The listing builds one solid part. Answer for the finished solid, in the listing's coordinates (mm). A direction names the side the tool comes from. Give positions to 0.01 mm unless a question says otherwise; leave off trailing zeros. Order: outer loops, then holes, each group sorted by start corner. A loop starts at its lowest first (then second) coordinate and runs counter-clockwise, first axis right, second up. Notation, with made-up numbers: (31.25, 76) - (68.25, 76) arc R15 ccw to (68.25, 87) - close; hole circle Ø5 at (1.5, -20). An arc over 180 degrees is marked (long way). Answer in a Markdown table with one row per item. Add a question column.
```python
from build123d import *

# Parameters (mm, degrees)
SKETCH1_W                                        = 22.225
SKETCH1_H                                        = 25.4
EXTRUDE1_DEPTH                                   = 12.7
SKETCH2_W                                        = 9.525
SKETCH2_H                                        = 0.762
EXTRUDE2_DEPTH                                   = 25.4
SKETCH3_W                                        = 0.762
SKETCH3_H                                        = 13.678822609
EXTRUDE3_DEPTH                                   = 25.4
EXTRUDE4_DEPTH                                   = 25.4
SKETCH7_W                                        = 3.175
SKETCH7_H                                        = 25.4
EXTRUDE5_DEPTH                                   = 6.74624
SKETCH8_W                                        = 15.875
SKETCH8_H                                        = 15.875
EXTRUDE6_DEPTH                                   = 25.4
F_1_4_20_TAPPED_HOLE1_D                          = 5.1054
F_1_4_20_TAPPED_HOLE1_DEPTH                      = 9.525
F_1_4_20_TAPPED_HOLE1_TIP                        = 1.533816902
EXTRUDE7_DEPTH                                   = 53.055785583
SKETCH10_W                                       = 9.525
SKETCH10_H                                       = 7.700729076
EXTRUDE8_DEPTH                                   = 25.4
CBORE_FOR_1_4_SOCKET_HEAD_CAP_SCREW1_D           = 6.7564
CBORE_FOR_1_4_SOCKET_HEAD_CAP_SCREW1_DEPTH       = 9.525
CBORE_FOR_1_4_SOCKET_HEAD_CAP_SCREW1_CBORE_D     = 11.1125
CBORE_FOR_1_4_SOCKET_HEAD_CAP_SCREW1_CBORE_DEPTH = 6.35
F_1_4_20_TAPPED_HOLE2_D                          = 5.1054
FILLET1_R                                        = 1.5875
FILLET2_R                                        = 7.9375


with BuildPart() as part:
    # Sketch1 → Extrude1 (new, symmetric)
    with BuildSketch(Plane.XY):
        Rectangle(SKETCH1_W, SKETCH1_H)
        Polygon((0, 10.998522628), (-9.525, 5.499261314), (-9.525, -5.499261314), (0, -10.998522628), (9.525, -5.499261314), (9.525, 5.499261314), align=None, mode=Mode.SUBTRACT)
    extrude(amount=EXTRUDE1_DEPTH, both=True)

    # Sketch2 → Extrude2 (add)
    with BuildSketch(Plane.XY.offset(12.7)):
        with Locations((15.875, 5.969)):
            Rectangle(SKETCH2_W, SKETCH2_H)
        with Locations((15.875, -3.772822609)):
            Rectangle(SKETCH2_W, SKETCH2_H)
        with Locations((-15.875, -3.772822609)):
            Rectangle(SKETCH2_W, SKETCH2_H)
        with Locations((-15.875, 5.969)):
            Rectangle(SKETCH2_W, SKETCH2_H)
    extrude(amount=-EXTRUDE2_DEPTH)

    # Sketch3 → Extrude3 (add)
    with BuildSketch(Plane.XY.offset(12.7)):
        with Locations((21.0185, 2.685588695)):
            Rectangle(SKETCH3_W, SKETCH3_H)
        with Locations((-21.0185, 2.685588695)):
            Rectangle(SKETCH3_W, SKETCH3_H)
    extrude(amount=-EXTRUDE3_DEPTH)

    # Sketch4 → Extrude4 (add)
    with BuildSketch(Plane.XY.offset(12.7)):
        Polygon((-21.3995, 17.4625), (21.3995, 17.4625), (21.3995, 9.525), (14.2875, 9.525), (14.2875, 15.875), (-14.2875, 15.875), (-14.2875, 9.525), (-21.3995, 9.525), align=None)
    extrude(amount=-EXTRUDE4_DEPTH)

    # Sketch7 → Extrude5 (add)
    with BuildSketch(Plane(origin=(0, 17.4625, 0), x_dir=(1, 0, 0), z_dir=(0, 1, 0))):
        Rectangle(SKETCH7_W, SKETCH7_H)
    extrude(amount=EXTRUDE5_DEPTH)

    # Sketch8 → Extrude6 (add)
    with BuildSketch(Plane.XY.offset(12.7)):
        with Locations((0, 32.14624)):
            Rectangle(SKETCH8_W, SKETCH8_H)
    extrude(amount=-EXTRUDE6_DEPTH)

    # 1/4-20 Tapped Hole1
    with Locations(Plane(origin=(-10.978640872, 40.08374, -1.669383244), x_dir=(-1, 0, 0), z_dir=(0, 1, 0))):
        with Locations((-10.978640872, -6.268116756), (-10.978640872, 9.606883244)):
            Hole(F_1_4_20_TAPPED_HOLE1_D / 2, depth=F_1_4_20_TAPPED_HOLE1_DEPTH)
            with Locations((0, 0, -(F_1_4_20_TAPPED_HOLE1_DEPTH + F_1_4_20_TAPPED_HOLE1_TIP / 2))):  # 118° drill point
                Cone(0, F_1_4_20_TAPPED_HOLE1_D / 2, F_1_4_20_TAPPED_HOLE1_TIP, mode=Mode.SUBTRACT)

    # Sketch9 → Extrude7 (cut, through all)
    with BuildSketch(Plane.XY.offset(12.7)):
        Polygon((-1.5875, -10.081979076), (-1.5875, -12.7), (1.5875, -12.7), (1.5875, -10.081979076), (0, -10.998522628), align=None)
    extrude(amount=-EXTRUDE7_DEPTH, mode=Mode.SUBTRACT)

    # Sketch10 → Extrude8 (add)
    with BuildSketch(Plane.XY.offset(12.7)):
        with Locations((6.35, -16.550364538)):
            Rectangle(SKETCH10_W, SKETCH10_H)
        with Locations((-6.35, -16.550364538)):
            Rectangle(SKETCH10_W, SKETCH10_H)
    extrude(amount=-EXTRUDE8_DEPTH)

    # CBORE for 1/4 Socket Head Cap Screw1
    with Locations(Plane(origin=(11.1125, 0, 0), x_dir=(0, 0, -1), z_dir=(1, 0, 0))):
        with Locations((0, -14.2875)):
            CounterBoreHole(CBORE_FOR_1_4_SOCKET_HEAD_CAP_SCREW1_D / 2, CBORE_FOR_1_4_SOCKET_HEAD_CAP_SCREW1_CBORE_D / 2, CBORE_FOR_1_4_SOCKET_HEAD_CAP_SCREW1_CBORE_DEPTH, depth=CBORE_FOR_1_4_SOCKET_HEAD_CAP_SCREW1_DEPTH)

    # 1/4-20 Tapped Hole2 (through all)
    with Locations(Plane.ZY.offset(11.1125)):
        with Locations((0, -14.2875)):
            Hole(F_1_4_20_TAPPED_HOLE2_D / 2)

    # Fillet1
    fillet1_edges = [part.edges().sort_by_distance(p)[0] for p in [
        (-1.5875, 17.4625, 0),
        (1.5875, 17.4625, 0),
        (1.5875, 24.20874, 0),
        (-1.5875, 24.20874, 0),
        (11.1125, 5.588, 0),
        (20.6375, -3.391822609, 0),
        (-11.1125, -3.391822609, 0),
        (-11.1125, 5.588, 0),
        (20.6375, 5.588, 0),
        (11.1125, -3.391822609, 0),
        (-20.6375, -3.391822609, 0),
        (-20.6375, 6.35, 0),
        (-20.6375, 9.525, 0),
        (-20.6375, 5.588, 0),
        (9.525, -5.499261314, 0),
        (9.525, 5.499261314, 0),
        (0, 10.998522628, 0),
        (-9.525, 5.499261314, 0),
        (-9.525, -5.499261314, 0),
        (-11.1125, 6.35, 0),
        (-14.2875, 15.875, 0),
        (14.2875, 15.875, 0),
        (20.6375, 6.35, 0),
        (20.6375, 9.525, 0),
        (11.1125, 6.35, 0),
    ]]
    fillet(fillet1_edges, radius=FILLET1_R - 0.0001)  # a hair under: the kernel refuses the full size

    # Fillet2
    fillet2_edges = [part.edges().sort_by_distance(p)[0] for p in [
        (21.3995, 17.4625, 0),
        (-21.3995, 17.4625, 0),
    ]]
    fillet(fillet2_edges, radius=FILLET2_R)


solid = part.part
```
(1) Find section B-B, the plane z = 0. Give the number of separate pieces and of enclosed holes in the cut face, plus the area to 3 significant figures.
(2) The mould has two halves that part along Y. Classify faces 5 (the face through (4.818, 8.217, 0.178)), 6 (the face through (-16, -4.154, 0)), 7 (the face through (-19.01, 15.2, -0.18)): +Y half, -Y half, draft (parallel to the pull), parting line (faces both ways), or undercut.
(3) Find section A-A, the plane x = 7. Write down the section's boundary in (y, z) (1 decimal), plus the area to 3 significant figures.
(4) Find section C-C, the plane y = -13.5. Write down the section's boundary in (x, z), plus the area to 3 significant figures.
(5) Straight lines are drawn through the part: line 1 (X direction, y = 2, z = 0.75) (1 decimal); line 2 (Y direction, x = -12.5, z = -2.75) (1 decimal); line 3 (Z direction, x = 0, y = 36.5). For each, find the intervals that lie inside material, in ascending order.
(6) For faces 1 (the face through (-8, 17.462, 0)), 2 (the face through (20.16, 9.07, -0.18)), 3 (the face through (6, 24.209, 0)), 4 (the face through (7.98, -12.62, -5.3)), determine the directions among +Z, -Z, +X, -X, +Y, -Y from which every point of the face is accessible in a straight line to the end or side of a thin tool.
(7) Each of these flat-tipped pins is pushed along its axis until it touches: P1, Ø9, axis at y = -14.29, z = 0, coming from the +X side; P2, Ø5, axis at y = 31.5, z = -3.5, coming from the -X side; P3, Ø11.5, axis at x = 18.5, z = -4.5, coming from the -Y side. Where does it stop, or does it pass through?
(8) Find section D-D, the plane x = 15.5. Write down the section's boundary in (y, z) (3 decimals), plus the area to 3 significant figures.
Answer key:
| question | item | result |
|---|---|---|
| 1 | separate pieces | 3 |
| 1 | enclosed holes | 3 |
| 1 | area | 715 mm² |
| 2 | face 5 | undercut |
| 2 | face 6 | -Y half |
| 2 | face 7 | +Y half |
| 3 | outline | (-20.4, -12.7) - (-7, -12.7) - (-7, 12.7) - (-20.4, 12.7) - close; (7, -12.7) - (12.7, -12.7) - (12.7, 12.7) - (7, 12.7) - close; (15.9, -12.7) - (17.5, -12.7) - (17.5, 12.7) - (15.9, 12.7) - close; (24.2, -12.7) - (40.1, -12.7) - (40.1, 12.7) - (24.2, 12.7) - close; hole circle Ø11.1 at (-14.3, 0) |
| 3 | area | 834 mm² |
| 4 | outline | (-11.11, -12.7) - (-1.59, -12.7) - (-1.59, -2.43) - (-11.11, -2.43) - close; (-11.11, 2.43) - (-1.59, 2.43) - (-1.59, 12.7) - (-11.11, 12.7) - close; (1.59, -12.7) - (11.11, -12.7) - (11.11, -5.5) - (4.76, -5.5) - (4.76, -3.29) - (1.59, -3.29) - close; (1.59, 3.29) - (4.76, 3.29) - (4.76, 5.5) - (11.11, 5.5) - (11.11, 12.7) - (1.59, 12.7) - close |
| 4 | area | 347 mm² |
| 5 | line 1 | -21.4 to -20.6, -11.1 to -9.5, 9.5 to 11.1, 20.6 to 21.4 |
| 5 | line 2 | -4.2 to -3.4, 5.6 to 6.4, 15.9 to 17.5 |
| 5 | line 3 | -12.7 to -10.49, -5.38 to 5.38, 10.49 to 12.7 |
| 6 | face 1 | +Z, -Z, -X |
| 6 | face 2 | +Z, -Z |
| 6 | face 3 | +Z, -Z, +X |
| 6 | face 4 | +X |
| 7 | P1 | x = 4.76 |
| 7 | P2 | x = -7.94 |
| 7 | P3 | y = -4.15 |
| 8 | outline | (-4.154, -12.7) - (-3.392, -12.7) - (-3.392, 12.7) - (-4.154, 12.7) - close; (5.588, -12.7) - (6.35, -12.7) - (6.35, 12.7) - (5.588, 12.7) - close; (9.525, -12.7) - (17.196, -12.7) - (17.196, 12.7) - (9.525, 12.7) - close |
| 8 | area | 234 mm² |
